Geometry: see drawing. Coordinates: mm, zero at the bounding-box minimum. Give positions to 0.01 mm unless a question says otherwise; leave off trailing zeros. Write each loop counter-clockwise with the first axis right and the second up, starting at its lowest first coordinate (ties: lowest second). Pieces come first, ordered by that corner, then holes. Notation, with made-up numbers: M 6.5,60 L 57.5,60 A13 ccw 57.5,82 Z; hole C -25.75,4 d6. An arc over 180 degrees is marked long. Answer as a JSON object with one key per item and string values. Group by question number.
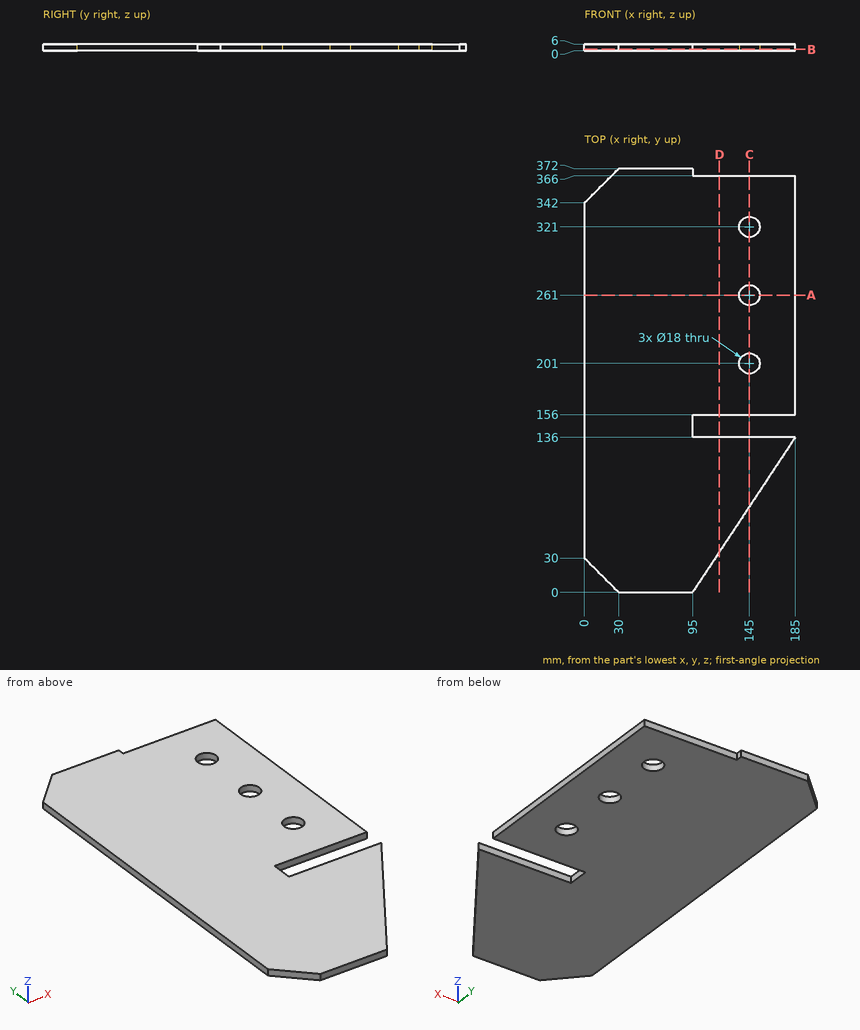
(1) Section D-D, the plane x = 118.5. Return loops of the section in (y, z), plus the area to 3 significant figures.
(2) Contact query for flat-ended pins moving along their axis: pin 1 Ø20.5 at (x, y) = (145, 321) entering from +Z; pin 2 Ø3 at (y, z) = (141.5, 4) entering from +X; pin 3 Ø1.8 at (x, z) = (137.5, 2) entering from -Y. Output: stop coordinate, or through.
(3) Section C-C, the plane x = 145. Return loops of the section in (y, z).
(4) Section B-B, the plane z = 1.2. Return loops of the section in (x, y), plus the area to 3 significant figures.
(5) Section A-A, the plane y = 261. Return loops of the section in (x, z).
(6) Ray query, L1, parallel to X at y = 201, z = 1.5; L2, parallel to Y at x = 145, z = 1.4; L3, parallel to Y at x = 150.5, z = 3.15. Return the intervals inside material, ascending. Write a range as [from, to].
Reported:
{
 "1": {"outline": "M 35.51,0 L 136,0 L 136,6 L 35.51,6 Z; M 156,0 L 366,0 L 366,6 L 156,6 Z", "area": "1,860 mm2"},
 "2": {"pin 1": "stops at z = 6", "pin 2": "stops at x = 95", "pin 3": "stops at y = 62.86"},
 "3": {"outline": "M 75.56,0 L 136,0 L 136,6 L 75.56,6 Z; M 156,0 L 192,0 L 192,6 L 156,6 Z; M 210,0 L 252,0 L 252,6 L 210,6 Z; M 270,0 L 312,0 L 312,6 L 270,6 Z; M 330,0 L 366,0 L 366,6 L 330,6 Z"},
 "4": {"outline": "M 0,30 L 30,0 L 95,0 L 185,136 L 95,136 L 95,156 L 185,156 L 185,366 L 95,366 L 95,372 L 30,372 L 0,342 Z; hole C 145,201 d18; hole C 145,261 d18; hole C 145,321 d18", "area": "58,700 mm2"},
 "5": {"outline": "M 0,0 L 136,0 L 136,6 L 0,6 Z; M 154,0 L 185,0 L 185,6 L 154,6 Z"},
 "6": {"L1": "x = [0, 136], [154, 185]", "L2": "y = [75.56, 136], [156, 192], [210, 252], [270, 312], [330, 366]", "L3": "y = [83.87, 136], [156, 193.88], [208.12, 253.88], [268.12, 313.88], [328.12, 366]"}
}
